Answer from the drawing. Dimensions are ordinates in mm from the lowest x, y and z of the part. A direction names the side the tool comes from. Give positions to 0.01 mm unless a question says otherwise; leave off trailing zeros. Loops run counter-clockwise (first coordinate to the right, second up) from the corner with the lowest first, then second, coordinate; pieces in that order, holes last. Notation, with made-up numbers: (-7, 49.25) -> (23, 49.25) arc R13 ccw to (23, 70.25) -> close; hole circle Ø7 at (52, 41). An arc over 180 degrees is marked (long way). Write each question's results on one line, items separated by ' | '. Start each with the question number.
Item 1: Section B-B on z = 4 is taken. State how many separate pieces and enclosed holes the cut face has, and give its area (3 significant figures).
Item 2: Each of these flat-tipped pins is pushed along its axis until it touches: P1, Ø12, axis at y = 24.5, z = 15.5, coming from the +X side (1 decimal); P2, Ø3, axis at x = 30, y = 29.5, coming from the +Z side; P3, Ø10, axis at x = 18.5, z = 20.5, coming from the -Y side. Where does it stop, or does it pass through?
Item 3: Section D-D on z = 19.75 is taken. Write down the section's boundary in (x, y) (1 decimal).
Item 4: Determine the mould class of the marked faces 4, 5 and 6 for opening direction X: +X half, -X half, draft (parallel to the pull), parting line (faces both ways), or undercut.
Item 5: Which of the six approach directions +Z, -Z, +X, -X, +Y, -Y give full straight-line access (tool end or side, diameter ignored) to the marked faces 1, 2 and 3?
Item 6: Find the intervals of material crossed by line 1 (X direction, y = 43.25, z = 19.05); line 2 (X direction, y = 7, z = 9.25) (1 decimal); line 3 (X direction, y = 23.5, z = 7), in increasing order.
Item 7: Section A-A on y = 8 is taken. Write down the section's boundary in (x, z) (1 decimal).
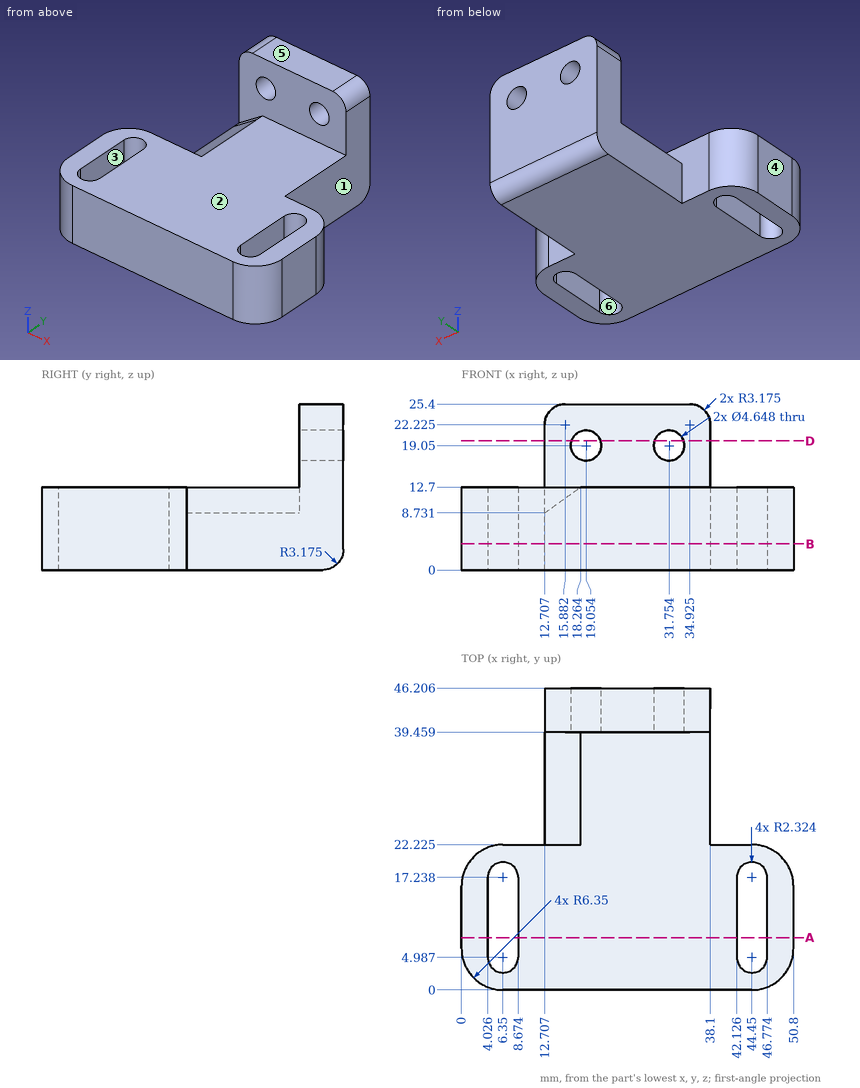
Findings:
1) separate pieces: 1 | enclosed holes: 2 | area: 1,560 mm2
2) P1: x = 49.9 | P2: z = 12.7 | P3: y = 39.46
3) outline: (12.7, 39.5) -> (16.8, 39.5) -> (16.8, 46.2) -> (12.7, 46.2) -> close; (21.3, 39.5) -> (29.5, 39.5) -> (29.5, 46.2) -> (21.3, 46.2) -> close; (34, 39.5) -> (38.1, 39.5) -> (38.1, 46.2) -> (34, 46.2) -> close
4) face 4: -X half | face 5: draft | face 6: undercut
5) face 1: +Z, -Z, +X, +Y | face 2: +Z, +X, -X, -Y | face 3: +Z, -Z
6) line 1: 12.71 to 16.73, 21.38 to 29.43, 34.08 to 38.1 | line 2: 0 to 4, 8.7 to 42.1, 46.8 to 50.8 | line 3: 12.71 to 38.1
7) outline: (0, 0) -> (4, 0) -> (4, 12.7) -> (0, 12.7) -> close; (8.7, 0) -> (42.1, 0) -> (42.1, 12.7) -> (8.7, 12.7) -> close; (46.8, 0) -> (50.8, 0) -> (50.8, 12.7) -> (46.8, 12.7) -> close
